Part model, mm, in its own coordinate system. Face numbers are marked on the shaded views. A direction names the side the tool comes from. Coordinates: 2 decimals unless noted, no trailing zeros. Loops run counter-clockwise (first coordinate to the right, second up) from the corner with the lowest first, then second, coordinate; pieces in that order, holes last. Notation, with made-up numbers: (-19, -19.5) - (6, -19.5) arc R23 ccw to (6, 8.5) - close; hole circle Ø4 at (12.25, -27). An arc over 180 degrees is marked (long way). Use a Markdown table: item, result. Add a question column.
1. Band-saw the part on B-B, the plane z = -5.75. Give the cut face in (x, y).
2. Band-saw the part on A-A, the plane x = 0. Give the cut face in (y, z).
3. 3-axis set-ups, long thin cutter, end or side, ignore diameter. For the marked faces 1 and 2: which of +Z, -Z, +X, -X, +Y, -Y reach the whole face in a straight line?
4. Band-saw the part on C-C, the plane y = 18.5. Give the cut face in (x, z), plus the area to 3 significant figures.
5. Wall check: probe 1 along X at (y, z) = (2.9, 0); probe 2 along Y at (x, z) = (3.5, -2.5); probe 3 along Y at (x, z) = (8.5, -1). Give the ranges that are in metal, low to high. Write a range as [from, to].
6. Band-saw the part on D-D, the plane z = 9.5. Give the cut face in (x, y), plus the area to 3 significant figures.
7. Drop flat-ended pins along their axis: pin 1 (0.9 mm diameter, centred on x = -8, z = 0.5, fed in from -Y); pin 2 (10 mm diameter, centred on x = 10, y = 14, fed in from +Z); pin 3 (5 mm diameter, centred on x = -4.5, z = 3.5, fed in from +Y). Give the stop position or say it passes through.
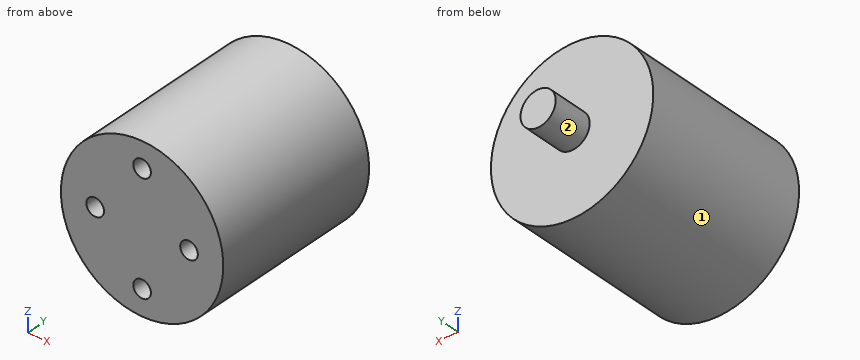
from build123d import *

# Parameters (mm, degrees)
SKETCH1_R           = 13.85
BOSS_EXTRUDE1_DEPTH = 30
SKETCH2_R           = 3
BOSS_EXTRUDE2_DEPTH = 7
SKETCH3_R           = 1.5
CUT_EXTRUDE1_DEPTH  = 4


with BuildPart() as part:
    # Sketch1 → Boss-Extrude1 (new body)
    with BuildSketch(Plane(origin=(0, 0, 0), x_dir=(1, 0, 0), z_dir=(0, 1, 0))):
        with Locations(Location((0, 0, 0), (0, 0, 270))):
            Circle(SKETCH1_R)
    extrude(amount=BOSS_EXTRUDE1_DEPTH)

    # Sketch2 → Boss-Extrude2 (add)
    with BuildSketch(Plane(origin=(0, 30, 0), x_dir=(1, 0, 0), z_dir=(0, 1, 0))):
        with Locations(Location((0, 0, 0), (0, 0, 270))):
            Circle(SKETCH2_R)
    extrude(amount=BOSS_EXTRUDE2_DEPTH)

    # Sketch3 → Cut-Extrude1 (cut)
    with BuildSketch(Plane(origin=(0, 0, 0), x_dir=(1, 0, 0), z_dir=(0, 1, 0))):
        with Locations(Location((8, 0, 0), (0, 0, 270))):
            Circle(SKETCH3_R)
        with Locations(Location((-8, 0, 0), (0, 0, 270))):
            Circle(SKETCH3_R)
        with Locations(Location((0, 9.5, 0), (0, 0, 270))):
            Circle(SKETCH3_R)
        with Locations(Location((0, -9.5, 0), (0, 0, 270))):
            Circle(SKETCH3_R)
    extrude(amount=CUT_EXTRUDE1_DEPTH, mode=Mode.SUBTRACT)


solid = part.part
Geometry check:
| question | item | result |
|---|---|---|
| 1 | outline | (-12.6, 0) - (12.6, 0) - (12.6, 30) - (-12.6, 30) - close |
| 2 | outline | (0, -13.85) - (30, -13.85) - (30, -3) - (37, -3) - (37, 3) - (30, 3) - (30, 13.85) - (0, 13.85) - (0, 11) - (4, 11) - (4, 8) - (0, 8) - (0, -8) - (4, -8) - (4, -11) - (0, -11) - close |
| 3 | face 1 | +Y, -Y |
| 3 | face 2 | +Y |
| 4 | outline | circle Ø27.7 at (0, 0) |
| 4 | area | 603 mm^2 |
| 5 | probe 1 | x = [-13.85, -9.5], [-6.5, 6.5], [9.5, 13.85] |
| 5 | probe 2 | y = [0, 30] |
| 5 | probe 3 | y = [4, 30] |
| 6 | outline | (-10.08, 0) - (-1.5, 0) - (-1.5, 4) - (1.5, 4) - (1.5, 0) - (10.08, 0) - (10.08, 30) - (-10.08, 30) - close |
| 6 | area | 593 mm^2 |
| 7 | pin 1 | stops at y = 4 |
| 7 | pin 2 | stops at z = 12.92 |
| 7 | pin 3 | stops at y = 30 |
